Here's how the part is built. I have some questions about the finished solid (model axes, mm). A direction names the side the tool comes from. Coordinates: 2 decimals unless noted, no trailing zeros. Order: outer loops, then holes, each group sorted by start corner. A loop starts at its lowest first (then second) coordinate and runs counter-clockwise, first axis right, second up. Notation, with made-up numbers: (-26, 46) - (-13, 46) arc R27 cw to (-13, 62) - close; hole circle Ø11 at (9, 50.25). An arc over 180 degrees is marked (long way). Answer in a Markdown table with one row per item. Add a question column.
Item 1: On a 3-axis mill with a long thin cutter (end or side, diameter ignored), from which of +Z, -Z, +X, -X, +Y, -Y can I reach the whole of each face in a straight line? I mean faces 4 (the flat face through (4, -8, 10.5)), 5 (the flat face through (4, 4, -13.5)), 6 (the flat face through (0, 3, -10.5)). Say none if no direction works.
Item 2: Will these pins go through, and if not, where does the flat tip stop? pin 1 Ø2 at (x, z) = (-4.5, -11) entering from -Y; pin 2 Ø6 at (x, y) = (1, 11.5) entering from -Z; pin 3 Ø3 at (x, z) = (13, -7) entering from +Y.
Item 3: I want a section at B-B (y = 0). Please give me the cut outline in (x, z).
Item 4: If I drill on line 1 along Y through (x, z) = (0, -18); line 2 along Z through (x, y) = (12.5, 2.5); line 3 along Y through (x, z) = (-14, 6.5), over which ranges is the centre line in solid material (lowest first)? Write a range as from..to.
Item 5: Thinking about a two-plate mould opening in Y: for faces 1 (the flat face through (0, 10, 0)), 2 (the flat face through (2.2, 2.2, -25)), 3 (the cylindrical face through (-1.08, 4.88, -19.17)), which applies, +Y half, -Y half, draft (parallel to the pull), parting line (faces both ways), or undercut?
Item 6: I want a section at C-C (z = 2.5). Please give me the cut outline in (x, y), plus the area to 3 significant figures.
Item 7: I want a section at D-D (x = -7). Please give me the cut outline in (y, z).
Item 8: I want a section at A-A (x = 0). Please give me the cut outline in (y, z), plus the area to 3 significant figures.
```python
from build123d import *

# Parameters (mm, degrees)
F0_R     = 17.5
F1_DEPTH = 10.5
F2_R     = 17.5
F3_DEPTH = 3
F4_R     = 5
F5_DEPTH = 11.5
F7_D     = 5.5
F7_DEPTH = 30
F7_TIP   = 1.6523667023


with BuildPart() as f1:
    # F0 (on Top) → F1 (new body, symmetric)
    with BuildSketch(Plane.XY):
        Circle(F0_R)
        with BuildLine():
            ThreePointArc((2.5, 7.5993420768), (0, -8), (-2.5, 7.5993420768))
            Line((-2.5, 7.5993420768), (-2.5, 10))
            Line((-2.5, 10), (2.5, 10))
            Line((2.5, 10), (2.5, 7.5993420768))
        make_face(mode=Mode.SUBTRACT)
    extrude(amount=F1_DEPTH, both=True)

    # F2 (on face) → F3 (join)
    with BuildSketch(Plane(origin=(0, 0, -10.5), x_dir=(1, 0, 0), z_dir=(0, 0, -1))):
        Circle(F2_R)
        with BuildLine():
            Line((-2.5, -10), (-2.5, -7.5993420768))
            ThreePointArc((-2.5, -7.5993420768), (0, 8), (2.5, -7.5993420768))
            Line((2.5, -7.5993420768), (2.5, -10))
            Line((2.5, -10), (-2.5, -10))
        make_face(mode=Mode.SUBTRACT)
        with BuildLine():
            ThreePointArc((2.5, -7.5993420768), (0, 8), (-2.5, -7.5993420768))
            Line((-2.5, -7.5993420768), (-2.5, -10))
            Line((-2.5, -10), (2.5, -10))
            Line((2.5, -10), (2.5, -7.5993420768))
        make_face()
    extrude(amount=F3_DEPTH)

    # F4 (on face) → F5 (join)
    with BuildSketch(Plane(origin=(0, 0, -13.5), x_dir=(1, 0, 0), z_dir=(0, 0, -1))):
        Circle(F4_R)
    extrude(amount=F5_DEPTH)

    # F7
    with Locations(Plane(origin=(0, 0, -25), x_dir=(1, 0, 0), z_dir=(0, 0, -1))):
        with Locations((0, 0)):
            Hole(F7_D / 2, depth=F7_DEPTH)
            with Locations((0, 0, -(F7_DEPTH + F7_TIP / 2))):  # 118° drill point
                Cone(0, F7_D / 2, F7_TIP, mode=Mode.SUBTRACT)


solid = f1.part
```
Values follow:
| question | item | result |
|---|---|---|
| 1 | face 4 | +Z, +X, -X, +Y, -Y |
| 1 | face 5 | -Z |
| 1 | face 6 | +Z |
| 2 | pin 1 | stops at y = -17.15 |
| 2 | pin 2 | stops at z = -13.5 |
| 2 | pin 3 | stops at y = 13.19 |
| 3 | outline | (-17.5, -13.5) - (-5, -13.5) - (-5, -25) - (-2.75, -25) - (-2.75, -10.5) - (-8, -10.5) - (-8, 10.5) - (-17.5, 10.5) - close; (2.75, -25) - (5, -25) - (5, -13.5) - (17.5, -13.5) - (17.5, 10.5) - (8, 10.5) - (8, -10.5) - (2.75, -10.5) - close |
| 4 | line 1 | y = -5..-2.75, 2.75..5 |
| 4 | line 2 | z = -13.5..10.5 |
| 4 | line 3 | y = -10.5..10.5 |
| 5 | face 1 | undercut |
| 5 | face 2 | draft |
| 5 | face 3 | parting line |
| 6 | outline | circle Ø35 at (0, 0); hole (-2.5, 7.6) arc R8 ccw (long way) to (2.5, 7.6) - (2.5, 10) - (-2.5, 10) - close |
| 6 | area | 750 mm^2 |
| 7 | outline | (-16.04, -13.5) - (16.04, -13.5) - (16.04, 10.5) - (3.87, 10.5) - (3.87, -10.5) - (-3.87, -10.5) - (-3.87, 10.5) - (-16.04, 10.5) - close |
| 8 | outline | (-17.5, -13.5) - (-5, -13.5) - (-5, -25) - (-2.75, -25) - (-2.75, -10.5) - (-8, -10.5) - (-8, 10.5) - (-17.5, 10.5) - close; (2.75, -25) - (5, -25) - (5, -13.5) - (17.5, -13.5) - (17.5, 10.5) - (10, 10.5) - (10, -10.5) - (2.75, -10.5) - close |
| 8 | area | 497 mm^2 |
